Here's how the part is built. I have some questions about the finished solid (model axes, mm). A direction names the side the tool comes from. Round coordinates to 2 decimals unless told otherwise and drop trailing zeros. Write each loop counter-clockwise with the first axis right and the second up, starting at its lowest first coordinate (ties: lowest second). Pieces come first, ordered by that corner, then holes. Notation, with made-up numbers: M 62,-17.75 L 118,-17.75 A25 cw 118,-2.75 Z; hole C 9,31 d5. An arc over 180 degrees is marked long. Write item = value, one per line. Start each with the question number.
(1) Will these pins go through, and if not, where does the flat tip stop? pin 1 Ø1.5 at (x, z) = (2, 6) entering from -Y; pin 2 Ø1 at (x, y) = (-2.5, 2) entering from +Z; pin 3 Ø5 at (x, y) = (4.5, -1.5) entering from +Z.
(2) I want a section at C-C (y = 0.5). List the corners of the cut face in (x, z) for me, and give its area (3 significant figures).
(3) I need wall thicknesses on line 1 along Z through (x, y) = (4.25, -0.5); line 2 along Z through (x, y) = (0, 0); line 3 along X through (y, z) = (-3.25, 1). Which ranges of each line are inside material? Lowest first, please.
(4) I want a section at D-D (x = 4.25). List the corners of the cut face in (y, z) for me, and give its area (3 significant figures).
(5) I want a section at B-B (x = -0.75). List the corners of the cut face in (y, z) for me.
(6) I want a section at A-A (z = 0.5). List the corners of the cut face in (x, y) for me, and give its area (3 significant figures).
(7) On a 3-axis mill with a long thin cutter (end or side, diameter ignored), from which of +Z, -Z, +X, -X, +Y, -Y can I reach the whole of each face in a straight line? I mean faces 1 (the flat face through (3, -3, 4)), 2 (the flat face through (-4.31, 2.535, 1.726)). Say none if no direction works.
```python
from build123d import *

# Parameters (mm, degrees)
F1_DEPTH = 4
F2_SIZE  = 0.5


with BuildPart() as f1:
    # F0 (on Top) → F1 (new body)
    with BuildSketch(Plane.XY):
        Polygon((2.886751, 5), (-2.886751, 5), (-5.773503, 0), (-2.886751, -5), (2.886751, -5), (5.773503, 0), align=None)
    extrude(amount=F1_DEPTH)

    # F2
    f2_edges = [f1.edges().sort_by_distance(p)[0] for p in [
        (4.330127, -2.5, 4),
        (0, -5, 4),
        (-4.330127, -2.5, 4),
        (-4.330127, 2.5, 4),
        (0, 5, 4),
        (4.330127, 2.5, 4),
    ]]
    chamfer(f2_edges, length=F2_SIZE)

    # F3 (on face) → F4 (revolve)
    with BuildSketch(Plane.XY.offset(4)):
        with BuildLine():
            Line((0, 4), (0, -4))
            ThreePointArc((0, -4), (4, 0), (0, 4))
        make_face()
    revolve(axis=Axis((0, 0, 4), (0, -1, 0)))


solid = f1.part
```
Returned:
q1.pin_1 = -3.42
q1.pin_2 = 6.95
q1.pin_3 = 7.31
q2.outline = M -5.48,0 L 5.48,0 L 5.48,3.5 L 4.91,4 L 3.97,4 A3.97 ccw -3.97,4 L -4.91,4 L -5.48,3.5 Z
q2.area = 68.3 mm²
q3.line_1 = 0 to 4
q3.line_2 = 0 to 8
q3.line_3 = -3.9 to 3.9
q4.outline = M -2.64,0 L 2.64,0 L 2.64,3.5 L 1.64,4 L -1.64,4 L -2.64,3.5 Z
q4.area = 20.6 mm²
q5.outline = M -5,0 L 5,0 L 5,3.5 L 4.5,4 L 3.93,4 A3.93 ccw -3.93,4 L -4.5,4 L -5,3.5 Z
q6.outline = M -5.77,0 L -2.89,-5 L 2.89,-5 L 5.77,0 L 2.89,5 L -2.89,5 Z
q6.area = 86.6 mm²
q7.face_1 = +Z
q7.face_2 = +Z, -Z, -X, +Y
